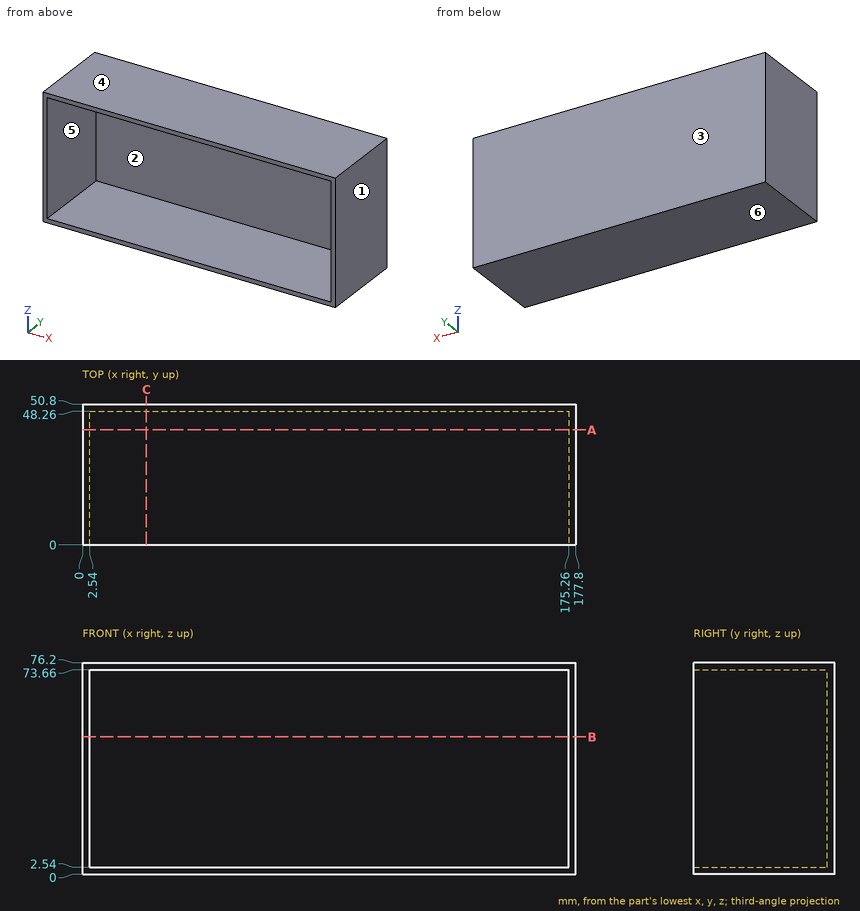
Job drawing, mm, ordinate dimensions from the low corner. One solid piece. A direction names the side the tool comes from. Coordinates: 2 decimals unless noted, no trailing zeros. Order: outer loops, then holes, each group sorted by start corner. A loop starts at its lowest first (then second) coordinate and runs counter-clockwise, first axis right, second up. Notation, with made-up numbers: (35, 56.5) - (57, 56.5) arc R22 cw to (57, 62.5) - close; hole circle Ø3 at (63.25, -16.5). An arc over 180 degrees is marked (long way). Write each question's results on one line, items separated by ' | '. Start each with the question number.
Item 1: Band-saw the part on A-A on y = 41.5. Write the cut outline in (x, z), and give its area (3 significant figures).
Item 2: Mould opens along Z. For the marked faces 3, 4, 5 and 6 say: released by +Z, released by -Z, zero draft, split by the parting line, or undercut.
Item 3: Tool access for the marked faces 1 and 2: list every direction of +Z, -Z, +X, -X, +Y, -Y with a clear straight run to the whole face (end or side of a thin tool).
Item 4: Wall check: probe 1 along X at (y, z) = (7, 10); probe 2 along Z at (x, y) = (43, 41.5); probe 3 along Y at (x, z) = (83.5, 17). Give the ranges that are in metal, low to high. Write a range as [from, to].
Item 5: Band-saw the part on B-B on z = 49.5. Write the cut outline in (x, y).
Item 6: Flat gauge pin, fed straight in: pin 1 (8 mm diameter, centred on x = 73.5, z = 56.5, fed in from -Y). Where does the tip first touch, or does it go through?
Item 7: Band-saw the part on C-C on x = 23. Write the cut outline in (y, z).
Numbers:
1) outline: (0, 0) - (177.8, 0) - (177.8, 76.2) - (0, 76.2) - close; hole (2.54, 2.54) - (175.26, 2.54) - (175.26, 73.66) - (2.54, 73.66) - close | area: 1,260 mm^2
2) face 3: zero draft | face 4: released by +Z | face 5: undercut | face 6: released by -Z
3) face 1: +Z, -Z, +X, +Y, -Y | face 2: -Y
4) probe 1: [0, 2.54], [175.26, 177.8] | probe 2: [0, 2.54], [73.66, 76.2] | probe 3: [48.26, 50.8]
5) outline: (0, 0) - (2.54, 0) - (2.54, 48.26) - (175.26, 48.26) - (175.26, 0) - (177.8, 0) - (177.8, 50.8) - (0, 50.8) - close
6) pin 1: y = 48.26
7) outline: (0, 0) - (50.8, 0) - (50.8, 76.2) - (0, 76.2) - (0, 73.66) - (48.26, 73.66) - (48.26, 2.54) - (0, 2.54) - close
